Autodesk Inventor part; units mm, degrees
ref_plane "YZ Plane" through (0, 0, 0) normal (1, 0, 0) x (0, 1, 0)
ref_plane "XZ Plane" through (0, 0, 0) normal (0, 1, 0) x (-1, 0, 0)
ref_plane "XY Plane" through (0, 0, 0) normal (0, 0, 1) x (1, 0, 0)
sketch "Sketch1" plane through (0, 0, 0) normal (0, 0, 1) x (1, 0, 0)
  line L0 (-40, -4) -> (40, -4)
  line L1 (40, -4) -> (40, 4)
  line L2 (40, 4) -> (-40, 4)
  line L3 (-40, 4) -> (-40, -4)
  line L4 (-40, -4) -> (40, 4) construction
  line L5 (40, -4) -> (-40, 4) construction
  point P0 (0, 0)
  dimension "d0" = 80
  dimension "d1" = 8
extrude "Extrusion1" add sketch "Sketch1" along normal blind 45
sketch "Sketch2" plane through (-40, 4, 0) normal (0, 1, 0) x (1, 0, 0)
  line L0 (80, -45) -> (0, -45)
  circle A0 centre (40, -45) radius 32
  point P0 (40, 0)
  dimension "d4" = 64
extrude "Extrusion2" cut sketch "Sketch2" against normal through all
ref_plane "Work Plane1" through (0, 0, 13.25) normal (0, 0, -1) x (-1, 0, 0)
sketch "Sketch3" plane through (0, 0, 13.25) normal (0, 0, -1) x (-1, 0, 0)
  point P0 (0, 0)
  point P1 (0, 0)
hole "Hole1" at (0, 0, 13.25) direction (0, 0, -1) diameter 3.4 end through all counterbore diameter 6.5 counterbore depth 3.4
sketch "Sketch4" plane through (0, 0, 45) normal (0, 0, 1) x (1, 0, 0)
  line L0 (40, -4) -> (40, 4)
  line L1 (-40, 4) -> (-40, -4)
  point P0 (0, 0)
  point P1 (36, 0)
  point P2 (-36, 0)
  dimension "d15" = 4
  dimension "d16" = 4
hole "Hole2" at (36, 0, 45) at (-36, 0, 45) direction (0, 0, -1) diameter 3.4 depth 12 tip angle 118
properties part number "Cap_Holder_1"
Work out the finished part from the listing and answer in its coordinate system (mm). A direction names the side the tool comes from. Round coordinates to 2 decimals unless told otherwise and drop trailing zeros. Loops run counter-clockwise (first coordinate to the right, second up) from the corner with the lowest first, then second, coordinate; pieces in that order, holes last. Notation, with made-up numbers: M 76,-20.75 L 87,-20.75 A14 cw 87,-16.75 Z; hole C 2.5,-3.75 d9. An arc over 180 degrees is marked long. One line per question, with ' | ' between items. Start each with the question number.
(1) A cutting plane is placed at B-B on z = 20.5. Write down the section's boundary in (x, y).
(2) Flat-ended cylindrical pins translate along their axes: pin 1 Ø3 at (x, y) = (-17, -2.5) entering from +Z; pin 2 Ø3 at (x, y) = (-36, 0) entering from +Z; pin 3 Ø2 at (x, y) = (0, 0) entering from -Z; pin 4 Ø2 at (x, y) = (-1, 0.5) entering from +Z. Find the tip coordinate at first contact, or state that the pin passes through.
(3) A tool of negligible diameter and unlimited length cuts with its end or side. For faces 5 (the face through (-40, 0, 22)), 6 (the face through (1.978, 2.579, 11.485)), from which of +Z, -Z, +X, -X, +Y, -Y can it reach the whole face along a straight path? Write none if from no direction.
(4) A cutting plane is placed at D-D on y = 2.5. Write down the section's boundary in (x, z).
(5) A cutting plane is placed at A-A on z = 35. Write down the section's boundary in (x, y).
(6) For a pull along Y with two mould halves and no side action, classify faces 1 (the face through (-1, -4, 12)), 2 (the face through (1.4, -1.4, 9.85)), 3 (the face through (1, 4, 12)), 4 (the face through (34, 0, 45)) as released by +Y, released by -Y, zero draft, split by the parting line, or undercut.
(7) A cutting plane is placed at C-C on z = 11. Write down the section's boundary in (x, y).
(8) Find the intervals of material crossed by line 1 (X direction, y = 0, z = 36.75); line 2 (Y direction, x = -36, z = 42.25); line 3 (Y direction, x = 0, z = 11), in increasing order.
Geometry check:
1) outline: M -40,-4 L -20.59,-4 L -20.59,4 L -40,4 Z; M 20.59,-4 L 40,-4 L 40,4 L 20.59,4 Z
2) pin 1: stops at z = 18.89 | pin 2: stops at z = 32.88 | pin 3: passes through | pin 4: stops at z = 9.85
3) face 5: +Z, -Z, -X, +Y, -Y | face 6: +Z
4) outline: M -40,0 L 40,0 L 40,45 L 32,45 A32 cw 2.08,13.07 L 2.08,9.85 L -2.08,9.85 L -2.08,13.07 A32 cw -32,45 L -40,45 Z
5) outline: M -40,-4 L -30.4,-4 L -30.4,4 L -40,4 Z; M 30.4,-4 L 40,-4 L 40,4 L 30.4,4 Z; hole C -36,0 d3.4; hole C 36,0 d3.4
6) face 1: released by -Y | face 2: undercut | face 3: released by +Y | face 4: zero draft
7) outline: M -40,-4 L 40,-4 L 40,4 L -40,4 Z; hole C 0,0 d6.5
8) line 1: x = -40 to -37.7, -34.3 to -30.92, 30.92 to 34.3, 37.7 to 40 | line 2: y = -4 to -1.7, 1.7 to 4 | line 3: y = -4 to -3.25, 3.25 to 4
